For this review, use the dimensioned drawing (mm, ordinates from the lowest corner) and the shaded views. A direction names the side the tool comes from. Coordinates: 2 decimals unless noted, no trailing zeros. Write each loop counter-clockwise with the first axis right and the second up, starting at its lowest first coordinate (ties: lowest second). Pieces come first, ordered by that corner, then holes. Notation, with made-up numbers: (58, 27.25) - (112, 27.25) arc R35 ccw to (112, 65.25) - close; hole circle Ø4 at (-19.5, 82). An arc over 180 degrees is marked (long way). Answer as a JSON object with one key per item and string values.
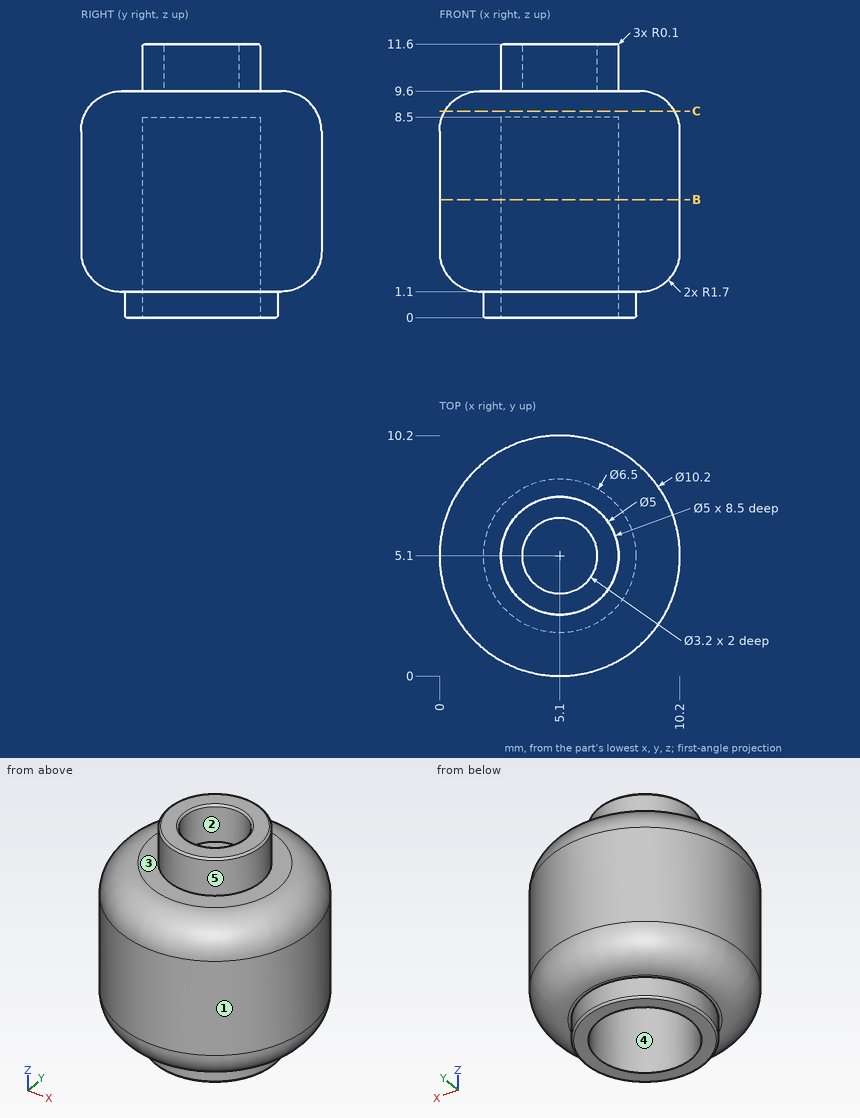
(1) Take a section at C-C, the plane z = 8.75. Write out the cut boundary in (x, y), and give its area (3 significant figures).
Solved:
{"outline": "circle Ø9.74 at (5.1, 5.1)", "area": "74.6 mm^2"}
(2) Tool access review of the marked faces 4 and 5: name each direction out of +Z, -Z, +X, -X, +Y, -Y from which nothing blocks a thin tool from reaching the whole face with its end or side.
Solved:
{"face 4": "-Z", "face 5": "+Z"}
(3) The part is to be moulded in two halves that separate along Y. For the marked faces 1, 2 and 3, say which applies: pulls with the +Y half, pulls with the -Y half, needs draft (parallel to the pull), parting line crosses it, or undercut.
Solved:
{"face 1": "parting line crosses it", "face 2": "undercut", "face 3": "needs draft"}
(4) Take a section at B-B, the plane z = 5. Write out the cut boundary in (x, y), and give its area (3 significant figures).
Solved:
{"outline": "circle Ø10.2 at (5.1, 5.1); hole circle Ø5 at (5.1, 5.1)", "area": "62.1 mm^2"}
(5) For pin 1 (1.5 mm diameter, centred on x = 4, z = 7, fed in from +Y); pin 2 (2 mm diameter, centred on y = 6.5, z = 9, fed in from +X); pin 3 (1.6 mm diameter, centred on x = 5.5, y = 4.5, fed in from +Z), all flat-tipped, find the tip position at first contact; note any pin that passes through.
Solved:
{"pin 1": "stops at y = 10.19", "pin 2": "stops at x = 10.11", "pin 3": "stops at z = 9.6"}
(6) To check wall thickness, follow line 1 (X direction, y = 5.25, z = 4); line 2 (Y direction, x = 5.1, z = 10.35). State the ranges of each line that lie inside material, in increasing order. Write a range as from..to.
Solved:
{"line 1": "x = 0..2.6, 7.6..10.2", "line 2": "y = 2.6..3.5, 6.7..7.6"}
